Model file for the job. Use its own axes, mm. Coordinates: 2 decimals unless noted, no trailing zeros. Loops run counter-clockwise (first coordinate to the right, second up) from the corner with the lowest first, then second, coordinate; pieces in that order, holes last. Notation, with made-up numbers: M 11.5,-6.75 L 49.5,-6.75 A34 cw 49.5,23.25 Z; hole C 64.25,82 d11. An arc over 180 degrees is marked long. Write item = value, one per line. Start each with the question number.
from build123d import *

# Parameters (mm, degrees)
BOSS_EXTRUDE1_DEPTH = 8.89
FILLET1_R           = 8.89
SKETCH4_R           = 25.4
SKETCH11_R          = 15.875


with BuildPart() as part:
    # Sketch1 → Boss-Extrude1 (new body)
    with BuildSketch(Plane(origin=(0, 0, 0), x_dir=(1, 0, 0), z_dir=(0, 1, 0))):
        with BuildLine():
            Line((0, 0), (63.5, 0))
            Line((63.5, 0), (63.5, 50.8))
            Line((63.5, 50.8), (0, 50.8))
            ThreePointArc((0, 50.8), (-25.4, 25.4), (0, 0))
        make_face()
    extrude(amount=BOSS_EXTRUDE1_DEPTH)

    # Fillet1
    fillet1_edges = [part.edges().sort_by_distance(p)[0] for p in [
        (63.5, 4.445, -50.8),
        (63.5, 4.445, 0),
    ]]
    fillet(fillet1_edges, radius=FILLET1_R)

    # Sketch4 → Loft2 section 0
    with BuildSketch(Plane(origin=(0, 8.89, 0), x_dir=(1, 0, 0), z_dir=(0, 1, 0))):
        with Locations((0, 25.4)):
            Circle(SKETCH4_R)
    # Sketch11 → Loft2 section 1
    with BuildSketch(Plane(origin=(0, 24.13, 0), x_dir=(1, 0, 0), z_dir=(0, 1, 0))):
        with Locations((0, 25.4)):
            Circle(SKETCH11_R)
    loft()


solid = part.part
Item 1: Cut at B-B (y = 10.5). Give the cut face in (x, z).
Item 2: Pin check, flat tip, straight feed: pin 1 Ø2 at (y, z) = (12, -10.5) entering from -X. Stop position of the tip, or through.
Item 3: Cut at A-A (x = 43). Give the cut face in (y, z).
Item 4: Cut at C-C (y = 21.75). Give the cut face in (x, z) (1 decimal), plus the area to 3 significant figures.
Item 5: Probe L1, parallel to Y at x = 41, z = -35; L2, parallel to X at y = 1.5, z = -25; L3, parallel to Z at x = 59, y = 1.5. List the from-to ranges inside material, lowest first.
Reported:
q1.outline = C 0,-25.4 d48.79
q2.pin_1 = -19.23
q3.outline = M 0,-50.8 L 8.89,-50.8 L 8.89,0 L 0,0 Z
q4.outline = C 0,-25.4 d34.7
q4.area = 947 mm^2
q5.L1 = 0 to 8.89
q5.L2 = -25.4 to 63.5
q5.L3 = -49.64 to -1.16
